Model file for the job. Use its own axes, mm. A direction names the side the tool comes from. Round coordinates to 2 decimals unless told otherwise and drop trailing zeros. Order: outer loops, then holes, each group sorted by start corner. A loop starts at its lowest first (then second) coordinate and runs counter-clockwise, first axis right, second up. Notation, with made-up numbers: (75.25, 18.5) - (90.25, 18.5) arc R23 cw to (90.25, 44.5) - close; hole circle Ø2 at (-20, -38.75). An arc over 180 degrees is marked (long way). Put each result on its own line as item: value. Start each with the question number.
Item 1: Mould opens along X. For faces 1 (the face through (1, 0, -17)), 2 (the face through (-28.56, -2.46, -12.84)) say: pulls with the +X half, pulls with the -X half, needs draft (parallel to the pull), parting line crosses it, or undercut.
Item 2: Saw through at A-A on y = -1.25. List the corners of the cut face in (x, z) (3 decimals).
Item 3: Saw through at B-B on x = 9. List the corners of the cut face in (y, z), plus the area to 3 significant figures.
Item 4: Which spindle directions (+Z, -Z, +X, -X, +Y, -Y) get a long thin tool onto all of the face, cutting with end or side? Do faces 3 (the face through (-2.535, -4.93, -4.93)), 4 (the face through (5, -5, 0)), 5 (the face through (-10.56, -2.46, -12.84)), 6 (the face through (4, -3, -45)). Say none if no direction does.
Item 5: Pin check, flat tips, straight feed: pin 1 Ø1 at (y, z) = (-7, -3.5) entering from +X; pin 2 Ø2 at (x, z) = (26, -15.5) entering from +Y; pin 3 Ø3 at (y, z) = (-3.5, -6) entering from -X. Stop position of each tip, or through.
Item 6: Saw through at C-C on z = -29.5. List the corners of the cut face in (x, y), plus the area to 3 significant figures.
Item 7: Saw through at D-D on y = -6. List the corners of the cut face in (x, z), plus the area to 3 significant figures.
Item 8: Probe probe 1 along X at (y, z) = (-1.7, -29.5); probe 2 along Z at (x, y) = (-0.75, -2.7); probe 3 along X at (y, z) = (-3.3, -29.5). List the from-to ranges inside material, lowest first.
Autodesk Inventor part; units mm, degrees
ref_plane "YZ Plane" through (0, 0, 0) normal (1, 0, 0) x (0, 1, 0)
ref_plane "XZ Plane" through (0, 0, 0) normal (0, 1, 0) x (-1, 0, 0)
ref_plane "XY Plane" through (0, 0, 0) normal (0, 0, 1) x (1, 0, 0)
sketch "스케치1" plane through (0, 0, 0) normal (0, 1, 0) x (-1, 0, 0)
  line L0 (-10, 10) -> (10, 10)
  line L1 (10, 10) -> (10, -10)
  line L2 (10, -10) -> (-10, -10)
  line L3 (-10, -10) -> (-10, 10)
  line L4 (-10, 10) -> (10, -10) construction
  line L5 (10, 10) -> (-10, -10) construction
  line L6 (-10, -10) -> (-15, -10)
  line L7 (-15, -10) -> (-15, 10)
  line L8 (-15, 10) -> (-10, 10)
  line L9 (-10, 10) -> (-10, -10)
  circle A0 centre (0, 0) radius 45.75
  dimension "d0" = 20
  dimension "d1" = 20
  dimension "d2" = 5
  dimension "d17" = 91.5
ref_plane "작업 평면2" through (-10, 20, -10) normal (-1, 0, 0) x (0, 0, 1)
sketch "스케치2" plane through (-10, 20, -10) normal (-1, 0, 0) x (0, 0, 1)
  line L0 (20, -100) -> (20, 0)
  line L1 (0, 0) -> (20, 0)
  line L2 (0, 0) -> (0, -100)
  line L3 (20, -100) -> (0, -100)
  circle A0 centre (10, -91) radius 4.5
  point P0 (10, -20)
  dimension "d7" = 9
  dimension "d8" = 9
ref_plane "작업 평면1" through (-10, 20, 10) normal (0, 0, 1) x (1, 0, 0)
sketch "스케치3" plane through (-10, 20, 10) normal (0, 0, 1) x (1, 0, 0)
  line L0 (20, -20) -> (25, -20)
  line L1 (25, -20) -> (25, 0)
  line L2 (0, 0) -> (25, 0)
  line L3 (0, -100) -> (0, 0)
  line L4 (20, -100) -> (0, -100)
  line L5 (20, -20) -> (20, -100)
  line L6 (25, -20) -> (25, 0)
  line L7 (25, 0) -> (0, 0)
  arc A0 (25, -20) -> (20, 0) centre (-10.6945, -18.2986) ccw
  line L8 (20, 0) -> (25, 0)
  line L9 (25, 0) -> (25, -20)
  point P0 (10, -20)
  point P1 (20, 0)
  point P2 (25, -16.5972)
extrude "돌출4" [suppressed]
extrude "돌출5" [suppressed]
extrude "돌출6" add sketch "스케치1" against normal blind 10
ref_plane "작업 평면3" through (10, 0, -10) normal (0, 0, 1) x (1, 0, 0)
sketch "스케치4" plane through (10, 0, -10) normal (0, 0, 1) x (1, 0, 0)
  line L0 (0, -5) -> (-10, -5)
  line L1 (-10, -5) -> (-10, -80)
  line L2 (0, -80) -> (-10, -80)
  line L3 (0, -5) -> (0, -80)
  line L4 (-10, 0) -> (0, 0)
  line L5 (0, 0) -> (5, 0)
  line L6 (5, 0) -> (5, 3.4028)
  arc A0 (5, 3.4028) -> (0, 20) centre (-30.6945, 1.7014) ccw
  line L7 (-10, 20) -> (0, 20)
  line L8 (-10, 20) -> (-10, 0)
  line L9 (0, -5) -> (5, -5)
  line L10 (5, -5) -> (5, 0)
  line L11 (5, 0) -> (0, 0)
  line L12 (0, 0) -> (0, -5)
  line L13 (-55.75, -5) -> (35.75, -5)
  line L14 (-10, 0) -> (-15, 0)
  line L15 (-15, 0) -> (-15, -5)
  line L16 (-15, -5) -> (-10, -5)
  line L17 (-10, -5) -> (-10, 0)
  line L18 (-15, 0) -> (-10, -5)
  line L19 (0, 0) -> (5, -5)
  dimension "d20" = 5
sketch "스케치5" plane through (0, 0, 0) normal (0, 1, 0) x (1, 0, 0)
  circle A0 centre (0, 0) radius 45.75
  line L0 (15, -10) -> (-10, -10)
  line L1 (-10, 10) -> (15, 10)
  line L2 (-12.2866, 10.5) -> (15, 10.5)
  line L3 (15, 10.5) -> (15, -10.5)
  line L4 (15, -10.5) -> (-12.2866, -10.5)
  line L5 (-12.2866, -10.5) -> (-12.2866, 10.5)
  line L6 (15, 10) -> (15, -10)
  line L7 (-10, -10) -> (-10, 10)
  dimension "d22" = 0.5
extrude "돌출7" [suppressed]
sketch "스케치6" plane through (-12.2866, 0, -10.5) normal (0, 0, 1) x (1, 0, 0)
  line L0 (7.2866, 0) -> (12.2866, -5)
  line L1 (7.2866, 0) -> (7.2866, -5)
  line L2 (7.2866, -5) -> (12.2866, -5)
  line L3 (22.2866, 0) -> (27.2866, -5)
  line L4 (22.2866, 0) -> (22.2866, -5)
  line L5 (22.2866, -5) -> (27.2866, -5)
  point P0 (12.2866, 0)
extrude "돌출8" [suppressed]
extrude "돌출9" add sketch "스케치4" along normal blind 20.5 and the other way blind 0.5 contours L19 L5 L10
ref_plane "작업 평면4" through (-12.2866, -5, -10.5) normal (0, 0, 1) x (1, 0, 0)
sketch "스케치7" plane through (-12.2866, -5, -10.5) normal (0, 0, 1) x (1, 0, 0)
  line L0 (7.2866, 0) -> (7.2866, 5)
  line L1 (0, 5) -> (7.2866, 5)
  line L2 (0, 5) -> (0, 0)
  line L3 (7.2866, 0) -> (0, 0)
  line L4 (0, 5) -> (7.2866, 5)
  line L5 (7.2866, 5) -> (7.2866, 0)
  line L6 (7.2866, 0) -> (0, 0)
  line L7 (0, 0) -> (0, 5)
  point P0 (12.2866, 5)
extrude "돌출10" add sketch "스케치7" along normal blind 21
sketch "스케치8" plane through (-5, 0, -10) normal (0, 0, 1) x (1, 0, 0)
  line L0 (0, 0) -> (0, -5)
  line L1 (20, -10) -> (-5, -10)
  line L2 (20, -5) -> (15, 0)
  line L3 (0, 0) -> (15, 0)
  line L4 (0, 0) -> (5, 0)
  line L5 (5, 0) -> (5, -10)
  line L6 (5, -10) -> (0, -10)
  line L7 (0, -10) -> (0, 0)
  line L8 (0, 0) -> (5, -10)
  line L9 (0, -5) -> (-5, -5)
  line L10 (-5, -5) -> (-5, -10)
  line L11 (20, -5) -> (20, -10)
  dimension "d33" = 5
extrude "돌출11" add sketch "스케치8" along normal blind 21
sketch "스케치9" plane through (0, 0, 0) normal (0, 1, 0) x (1, 0, 0)
  line L0 (10, -10) -> (-10, -10)
  line L1 (10, 10) -> (10, -10)
  line L2 (64.05, 10) -> (-64.05, 10)
  line L3 (-10, -64.05) -> (-10, 64.05)
  line L4 (-10, -10) -> (-10, 10)
  line L5 (-10, 10) -> (10, 10)
  line L6 (10, -10) -> (0, -10)
  line L7 (0, -10) -> (0, 10)
  line L8 (0, 10) -> (10, 10)
  line L9 (10, 10) -> (10, -10)
  point P0 (0, 0)
extrude "돌출12" cut sketch "스케치9" against normal blind 10 contours L0 L7 L2 L1
sketch "스케치10" plane through (10, 0, 10) normal (0, 0, -1) x (-1, 0, 0)
  line L0 (-5, 0) -> (0, 0)
  line L1 (0, 0) -> (0, -10)
  line L2 (-35.75, -10) -> (55.75, -10)
  line L3 (0, 0) -> (-5, 0)
  line L4 (-5, 0) -> (-5, -10)
  line L5 (-5, -10) -> (0, -10)
  line L6 (0, -10) -> (0, 0)
  line L7 (0, 0) -> (-5, -10)
  line L8 (10, 0) -> (15, 0)
  line L9 (15, 0) -> (15, -10)
  line L10 (15, -10) -> (10, -10)
  line L11 (10, -10) -> (10, 0)
  line L12 (15, 0) -> (10, -10)
  dimension "d38" = 5
extrude "돌출13" cut sketch "스케치10" along normal blind 20 contours L11 L8 L12
extrude "돌출14" cut sketch "스케치10" along normal blind 20 contours L1 L2 L7
sketch "스케치11" plane through (10, 0, 10) normal (0, 0, -1) x (-1, 0, 0)
  line L0 (-35.75, -10) -> (55.75, -10)
  line L1 (55.75, 0) -> (-35.75, 0)
  line L2 (0, 0) -> (0, -10)
  line L3 (10, -10) -> (10, 0)
  line L4 (0, 0) -> (10, 0)
  line L5 (10, 0) -> (10, -10)
  line L6 (10, -10) -> (0, -10)
  line L7 (0, -10) -> (0, 0)
  circle A0 centre (5, -5) radius 2.5
  dimension "d43" = 5
extrude "돌출15" add sketch "스케치11" along normal blind 20 contours A0
sketch "스케치12" plane through (-10, 20, 10) normal (0, 0, 1) x (1, 0, 0)
  point P0 (10, -20)
sketch "스케치13" plane through (0, 0, 0) normal (0, 0, 1) x (1, 0, 0)
  line L0 (-45.75, -10) -> (45.75, -10)
  line L1 (45.75, 0) -> (-45.75, 0)
  line L2 (-45.75, -10) -> (45.75, -10)
  line L3 (-45.75, 0) -> (45.75, 0)
  line L4 (45.75, 0) -> (45.75, -10)
  line L5 (45.75, -10) -> (-45.75, -10)
  line L6 (-45.75, -10) -> (-45.75, 0)
  point P0 (0, 0)
extrude "돌출16" cut sketch "스케치13" along normal blind 50
sketch "스케치14" plane through (0, 0, 0) normal (0, 0, 1) x (1, 0, 0)
  line L0 (-38.75, -7) -> (-13.75, -7)
  line L1 (-13.75, -7) -> (-13.75, -3)
  line L2 (-13.75, -3) -> (-38.75, -3)
  line L3 (-38.75, -3) -> (-38.75, -7)
  line L4 (0, -10) -> (-45.75, -10)
  line L5 (-45.75, 0) -> (-45.75, -10)
  circle A0 centre (5, -5) radius 2.5
  line L6 (5, -26.6285) -> (5, 24.5755)
  line L7 (21, -7) -> (41, -7)
  line L8 (41, -7) -> (41, -3)
  line L9 (41, -3) -> (21, -3)
  line L10 (21, -3) -> (21, -7)
  line L11 (45.75, 0) -> (45.75, -10)
  line L12 (-45.75, -3) -> (-44.55, -3)
  line L13 (-44.55, -3) -> (-44.55, -7)
  line L14 (-44.55, -7) -> (-45.75, -7)
  line L15 (-45.75, -7) -> (-45.75, -3)
  line L16 (0, -36.8693) -> (0, 34.8163)
  point P0 (0, 0)
  point P1 (45.75, -5)
  dimension "d48" = 25
  dimension "d49" = 4
  dimension "d50" = 3
  dimension "d51" = 7
  dimension "d52" = 20
  dimension "d53" = 4
  dimension "d54" = 4.75
  dimension "d57" = 1.2
extrude "돌출17" add sketch "스케치14" along normal blind 5 contours L3 L2 L1 L0 | L10 L9 L8 L7
revolve "회전1" cut sketch "스케치14" angle 360 about axis through (0, -10, 0) along (0, 1, 0) contours L12 L13 L14 L5
sketch "스케치15" plane through (0, 0, 0) normal (0, 1, 0) x (1, 0, 0)
  circle A0 centre (-27.75, 16.5) radius 3.75
  circle A1 centre (-9.75, 16.5) radius 3.75
  circle A2 centre (8.25, 16.5) radius 3.75
  circle A3 centre (26.25, 16.5) radius 3.75
  circle A4 centre (-18.75, 29.5) radius 3.75
  circle A5 centre (-0.75, 29.5) radius 3.75
  line L0 (-44.55, 0) -> (-45.75, 0)
  line L1 (-45.75, 0) -> (-45.75, 37.0208)
  circle A6 centre (17.25, 29.5) radius 3.75
  line L2 (64.05, 10.5) -> (-64.05, 10.5)
  point P0 (0, 0)
  dimension "d59" = 7.5
  dimension "d60" = 7.5
  dimension "d61" = 7.5
  dimension "d62" = 7.5
  dimension "d63" = 7.5
  dimension "d64" = 7.5
  dimension "d66" = 18
  dimension "d67" = 18
  dimension "d68" = 18
  dimension "d69" = 18
  dimension "d70" = 9
  dimension "d71" = 9
  dimension "d73" = 7.5
  dimension "d74" = 9
  dimension "d75" = 13
  dimension "d76" = 13
  dimension "d77" = 13
  dimension "d80" = 6
  dimension "d81" = 6
extrude "돌출18" cut sketch "스케치15" against normal blind 5
properties part number "new탄두윗판구멍1_1_3"
Results found:
1. face 1: needs draft
1. face 2: undercut
2. outline: (-45.75, 0) arc R45.75 ccw to (45.75, 0) - (10.625, 0) - (10.625, -10) - (-4.375, -10) - (-4.375, 0) - close; hole circle Ø7.5 at (-27.75, -16.5); hole circle Ø7.5 at (-18.75, -29.5); hole circle Ø7.5 at (-9.75, -16.5); hole circle Ø7.5 at (-0.75, -29.5); hole circle Ø7.5 at (8.25, -16.5); hole circle Ø7.5 at (17.25, -29.5); hole circle Ø7.5 at (26.25, -16.5)
3. outline: (-10, -44.86) - (-7, -44.86) - (-7, -43.63) - (-3, -43.63) - (-3, -44.86) - (0, -44.86) - (0, -20.17) - (-5, -20.17) - (-5, -12.83) - (0, -12.83) - (0, -10) - (-10, -10) - close
3. area: 307 mm²
4. face 3: +Z, +Y
4. face 4: +Z, +Y, -Y
4. face 5: +Y
4. face 6: -Z
5. pin 1: stops at x = 45.65
5. pin 2: stops at y = -5
5. pin 3: stops at x = -45.52
6. outline: (-34.97, -10) - (34.97, -10) - (34.97, -7) - (33.38, -7) - (33.38, -3) - (34.97, -3) - (34.97, 0) - (21, 0) - (21, -5) - (13.5, -5) - (13.5, 0) - (3, 0) - (3, -5) - (-4.5, -5) - (-4.5, 0) - (-15, 0) - (-15, -5) - (-22.5, -5) - (-22.5, 0) - (-34.97, 0) - (-34.97, -3) - (-33.38, -3) - (-33.38, -7) - (-34.97, -7) - close
6. area: 574 mm²
7. outline: (-44.55, 0) arc R44.55 ccw to (44.55, 0) - (41, 0) - (41, 5) - (21, 5) - (21, 0) - (13, 0) - (13, -10) - (7.29, -10) - (7.29, 0) - (2.71, 0) - (2.71, -10) - (-2, -10) - (-2, 0) - (-13.75, 0) - (-13.75, 5) - (-38.75, 5) - (-38.75, 0) - close
7. area: 3,240 mm²
8. probe 1: x = -34.97 to -22.5, -15 to -4.5, 3 to 13.5, 21 to 34.97
8. probe 2: z = -45.74 to -33.25, -25.75 to -10
8. probe 3: x = -33.38 to -22.5, -15 to -4.5, 3 to 13.5, 21 to 33.38
